Input: part model. Units: mm. Frame: model coordinates. A direction names the side the tool comes from. Round coordinates to 2 decimals unless told otherwise and drop trailing zeros. Loops run counter-clockwise (first coordinate to the right, second up) from the corner with the lowest first, then second, coordinate; pieces in that order, holes last. Notation, with made-up numbers: (48, 62.25) -> (65, 62.25) arc R13 ccw to (65, 79.25) -> close; hole circle Ø10 at (25, 64). An arc over 180 degrees is marked (long way). Answer as a JSON object with one key per item and string values.
```python
from build123d import *

# Parameters (mm, degrees)
F3_DEPTH = 27.432
F5_DEPTH = 33.528


# Not quite as in the source:
# - the program builds the solid bodies; features that only make, move or delete a surface that nothing else refers to are left out


with BuildPart() as f3:
    # F2 (on Top) → F3 (new body)
    with BuildSketch(Plane.XY):
        with BuildLine():
            ThreePointArc((25.9753267238, -94.6690976426), (76.334874565, -60.3082301144), (95.7446020854, -2.515360713))
            ThreePointArc((95.7446020854, -2.515360713), (-57.7928694014, 73.819513852), (-25.9753267238, -94.6690976426))
            ThreePointArc((-25.9753267238, -94.6690976426), (0, -72.0376076224), (25.9753267238, -94.6690976426))
        make_face()
    extrude(amount=F3_DEPTH)

    # F4 (on face) → F5 (join)
    with BuildSketch(Plane.XY.offset(27.432)):
        with BuildLine():
            ThreePointArc((-55.0617836416, 75.8123407131), (-46.9138023818, 80.9479484388), (-38.2910855114, 85.23896453))
            Line((-38.2910855114, 85.23896453), (-38.2910855114, 107.650950551))
            Line((-38.2910855114, 107.650950551), (-55.0617836416, 107.650950551))
            Line((-55.0617836416, 107.650950551), (-55.0617836416, 75.8123407131))
        make_face()
        with BuildLine():
            Line((-55.0617836416, 0), (-38.2910855114, 0))
            Line((-38.2910855114, 0), (-38.2910855114, 85.23896453))
            ThreePointArc((-38.2910855114, 85.23896453), (-46.9138023818, 80.9479484388), (-55.0617836416, 75.8123407131))
            Line((-55.0617836416, 75.8123407131), (-55.0617836416, 0))
        make_face()
    extrude(amount=F5_DEPTH)


solid = f3.part
```
1) Reachability of faces 1 (the face through (-38.291, 53, 44)), 2 (the face through (-55.062, 55, 44)), 3 (the face through (-47, 95, 27.432)), 4 (the face through (-47, 0, 44)) from +Z, -Z, +X, -X, +Y, -Y: full face, straight path, thin tool, end or side. Return the list, or none.
Output:
{"face 1": "+Z, +X, +Y, -Y", "face 2": "+Z, -X, +Y, -Y", "face 3": "-Z, -X, +Y", "face 4": "+Z, +X, -X, -Y"}
2) Ray query, probe 1 along X at (y, z) = (-2, 14); probe 2 along Z at (x, y) = (-45, -45.5); probe 3 along X at (y, z) = (20.5, 47.5). Return the intervals inside material, ascending.
Output:
{"probe 1": "x = -95.74 to 95.74", "probe 2": "z = 0 to 27.43", "probe 3": "x = -55.06 to -38.29"}
3) Section C-C, the plane x = 0. Output: boundary loops of the cut face in (y, z).
Output:
{"outline": "(-72.04, 0) -> (93.23, 0) -> (93.23, 27.43) -> (-72.04, 27.43) -> close"}
4) Section A-A, the plane y = 63. Output: boundary loops of the cut face in (x, z).
Output:
{"outline": "(-69.82, 0) -> (69.82, 0) -> (69.82, 27.43) -> (-38.29, 27.43) -> (-38.29, 60.96) -> (-55.06, 60.96) -> (-55.06, 27.43) -> (-69.82, 27.43) -> close"}
5) Contact query for flat-ended pins moving along their axis: P1, Ø18.5, axis at x = -50.5, y = 90, coming from the -Z side; P2, Ø8, axis at x = -6, y = -52.5, coming from the +Z side; P3, Ø17, axis at y = 78.5, z = 38.5, coming from the -X side. Output: stop coordinate, or through.
Output:
{"P1": "stops at z = 27.43", "P2": "stops at z = 27.43", "P3": "stops at x = -55.06"}
6) Section D-D, the plane z = 52. Output: boundary loops of the cut face in (x, y).
Output:
{"outline": "(-55.06, 0) -> (-38.29, 0) -> (-38.29, 107.65) -> (-55.06, 107.65) -> close"}
7) Section B-B, the plane z = 21.5. Output: boundary loops of the cut face in (x, y), plus the area to 3 significant figures.
Output:
{"outline": "(-25.98, -94.67) arc R26.22 cw to (25.98, -94.67) arc R95.74 ccw (long way) to start", "area": "27,800 mm^2"}
